Build history of the part. All positions in model axes, mm. A direction names the side the tool comes from. Give positions to 0.01 mm unless a question says otherwise; leave off trailing zeros. Write each loop counter-clockwise with the first axis right and the second up, starting at its lowest first coordinate (ties: lowest second). Pieces come first, ordered by that corner, then holes.
from build123d import *

# Parameters (mm, degrees)
EXTRUDE_1_DEPTH      = 30
SKETCH_6_W           = 21.999074129
SKETCH_6_H           = 43.978081363
CUT_EXTRUDE_5_DEPTH  = 10
SKETCH_7_W           = 30
SKETCH_7_H           = 21.035862509
CUT_EXTRUDE_6_DEPTH  = 10
SKETCH_8_R           = 1.5
CUT_EXTRUDE_7_DEPTH  = 10
SKETCH_9_W           = 20
SKETCH_9_H           = 13.964137491
CUT_EXTRUDE_8_DEPTH  = 1
SKETCH_10_W          = 20
SKETCH_10_H          = 36
CUT_EXTRUDE_9_DEPTH  = 1
SKETCH_11_W          = 20
SKETCH_11_H          = 2
CUT_EXTRUDE_10_DEPTH = 8
SKETCH_12_R          = 2
CUT_EXTRUDE_11_DEPTH = 8


with BuildPart() as part:
    # 草图1 → 凸台-拉伸1 (new body)
    with BuildSketch(Plane(origin=(0, 0, 0), x_dir=(0, 0, -1), z_dir=(1, 0, 0))):
        Polygon((0, 0), (0, 35), (3, 35), (3, -3), (-35, -3), (-35, 0), align=None)
    extrude(amount=EXTRUDE_1_DEPTH)

    # 草图6 → 切除-拉伸5 (cut)
    with BuildSketch(Plane.ZY):
        with Locations((2.964600426, 15.968723176)):
            Rectangle(SKETCH_6_W, SKETCH_6_H)
    extrude(amount=-CUT_EXTRUDE_5_DEPTH, mode=Mode.SUBTRACT)

    # 草图7 → 切除-拉伸6 (cut)
    with BuildSketch(Plane(origin=(0, 0, 0), x_dir=(1, 0, 0), z_dir=(0, 1, 0))):
        with Locations((15, -24.482068746)):
            Rectangle(SKETCH_7_W, SKETCH_7_H)
    extrude(amount=-CUT_EXTRUDE_6_DEPTH, mode=Mode.SUBTRACT)

    # 草图8 → 切除-拉伸7 (cut)
    with BuildSketch(Plane(origin=(0, 0, 0), x_dir=(1, 0, 0), z_dir=(0, 1, 0))):
        with Locations((15, -6)):
            Circle(SKETCH_8_R)
        with Locations((25, -6)):
            Circle(SKETCH_8_R)
    extrude(amount=-CUT_EXTRUDE_7_DEPTH, mode=Mode.SUBTRACT)

    # 草图9 → 切除-拉伸8 (cut)
    with BuildSketch(Plane(origin=(0, 0, 0), x_dir=(1, 0, 0), z_dir=(0, 1, 0))):
        with Locations((20, -6.982068746)):
            Rectangle(SKETCH_9_W, SKETCH_9_H)
    extrude(amount=-CUT_EXTRUDE_8_DEPTH, mode=Mode.SUBTRACT)

    # 草图10 → 切除-拉伸9 (cut)
    with BuildSketch(Plane.XY):
        with Locations((20, 17)):
            Rectangle(SKETCH_10_W, SKETCH_10_H)
    extrude(amount=-CUT_EXTRUDE_9_DEPTH, mode=Mode.SUBTRACT)

    # 草图11 → 切除-拉伸10 (cut)
    with BuildSketch(Plane(origin=(0, 35, 0), x_dir=(1, 0, 0), z_dir=(0, 1, 0))):
        with Locations((20, 2)):
            Rectangle(SKETCH_11_W, SKETCH_11_H)
    extrude(amount=-CUT_EXTRUDE_10_DEPTH, mode=Mode.SUBTRACT)

    # 草图12 → 切除-拉伸11 (cut)
    with BuildSketch(Plane(origin=(0, 0, -3), x_dir=(-1, 0, 0), z_dir=(0, 0, -1))):
        with Locations((-20, 13)):
            Circle(SKETCH_12_R)
    extrude(amount=-CUT_EXTRUDE_11_DEPTH, mode=Mode.SUBTRACT)


solid = part.part
1. 3-axis set-ups, long thin cutter, end or side, ignore diameter. For faces 1 (the face through (20, -1, 6)), 2 (the face through (10, 7.6, -1.5)): which of +Z, -Z, +X, -X, +Y, -Y reach the whole face in a straight line?
2. Saw through at D-D on x = 20. Give the cut face in (y, z).
3. Mould opens along Y. For faces 3 (the face through (21.474, 14.352, -2.014)), 4 (the face through (20, -3, 5)), 5 (the face through (17.6, 13.2, -1)) say: pulls with the +Y half, pulls with the -Y half, needs draft (parallel to the pull), parting line crosses it, or undercut.
4. Saw through at A-A on z = 6. Give the cut face in (x, y), plus the area to 3 significant figures.
5. Saw through at B-B on x = 15. Give the cut face in (y, z).
6. Drill centre lines: line 1 along X through (y, z) = (-1.95, 6); line 2 along Y through (x, z) = (20, -1.55); line 3 along Z through (x, y) = (19.5, 19.25). Where is each one in solid material? Low to high.
7. Drop flat-ended pins along their axis: pin 1 (5 mm diameter, centred on x = 20.5, y = 13, fed in from +Z); pin 2 (2 mm diameter, centred on x = 15, z = 0.5, fed in from +Y). Give the stop position or say it passes through.
8. Saw through at C-C on y = 13. Give the cut face in (x, z).
Outcome:
1. face 1: +Z, +X, -X, +Y
1. face 2: +Z, -Z, -X, +Y, -Y
2. outline: (-3, -3) - (11, -3) - (11, -1) - (-1, -1) - (-1, 13.96) - (-3, 13.96) - close; (15, -3) - (27, -3) - (27, -1) - (15, -1) - close
3. face 3: undercut
3. face 4: pulls with the -Y half
3. face 5: needs draft
4. outline: (10, -3) - (13.5, -3) - (13.5, -1) - (10, -1) - close; (16.5, -3) - (23.5, -3) - (23.5, -1) - (16.5, -1) - close; (26.5, -3) - (30, -3) - (30, -1) - (26.5, -1) - close
4. area: 28.0 mm2
5. outline: (-3, -3) - (27, -3) - (27, -1) - (-1, -1) - (-1, 4.5) - (-3, 4.5) - close; (-3, 7.5) - (-1, 7.5) - (-1, 13.96) - (-3, 13.96) - close
6. line 1: x = 10 to 13.5, 16.5 to 23.5, 26.5 to 30
6. line 2: y = -3 to 11, 15 to 27
6. line 3: z = -3 to -1
7. pin 1: stops at z = -1
7. pin 2: stops at y = -1
8. outline: (10, -3) - (18, -3) - (18, -1) - (10, -1) - close; (22, -3) - (30, -3) - (30, -1) - (22, -1) - close
